Geometry check sheet. Reference: the model listing, model coordinates, mm. A direction names the side the tool comes from. Give positions to 0.01 mm unless a question says otherwise; leave off trailing zeros. Loops run counter-clockwise (first coordinate to the right, second up) from the corner with the lowest first, then second, coordinate; pieces in that order, holes last.
1. Cross-section at C-C, the plane x = 0. Record the cut outline in (y, z).
2. Material ranges on L1, parallel to X at y = 0.9, z = 0; L2, parallel to Z at x = -18.5, y = 0.9; L3, parallel to Y at x = -16, z = -0.5, recorded low to high.
3. Tool access check on faces 1 (the flat face through (-18, 1, 2.5)), 2 (the flat face through (22, 1, 0)), 3 (the flat face through (18, 1, -2.5)). Record the directions out of +Z, -Z, +X, -X, +Y, -Y that give a thin tool (end or side, any length) a straight path to the whole face; none if there is none.
4. Cross-section at A-A, the plane x = -18.5. Record the cut outline in (y, z).
5. Cross-section at D-D, the plane y = 8. Record the cut outline in (x, z).
6. Cross-section at B-B, the plane z = 0. Record the cut outline in (x, y), plus the area to 3 significant figures.
7. Go/stop test with flat-tipped pins: pin 1 Ø3.5 at (x, z) = (-2, -2.5) entering from +Y; pin 2 Ø2 at (x, y) = (-18, 0.5) entering from -Z; pin 3 Ø2 at (x, y) = (17.5, 0.5) entering from +Z. Record where each tip stops, or that it passes through.
8. Release check for a two-part mould opening along Y. For faces 4 (the cylindrical face through (-17.524, 0.986, 0.217)), 5 (the flat face through (0, 19, 0)) record: +Y half, -Y half, draft (parallel to the pull), parting line (faces both ways), or undercut.
from build123d import *

# Parameters (mm, degrees)
SKETCH1_W           = 30
SKETCH1_H           = 30
BOSS_EXTRUDE1_DEPTH = 6
FILLET1_R           = 10
SKETCH3_W           = 7
SKETCH3_H           = 5
SKETCH3_R           = 1
BOSS_EXTRUDE2_DEPTH = 2
FILLET3_R           = 1
SKETCH4_W           = 30
SKETCH4_H           = 30
BOSS_EXTRUDE3_DEPTH = 15
FILLET4_R           = 10
SKETCH5_R           = 5.5
CUT_EXTRUDE2_DEPTH  = 2


with BuildPart() as part:
    # Sketch1 → Boss-Extrude1 (new body)
    with BuildSketch(Plane(origin=(0, 0, 0), x_dir=(1, 0, 0), z_dir=(0, 1, 0))):
        Rectangle(SKETCH1_W, SKETCH1_H)
    extrude(amount=BOSS_EXTRUDE1_DEPTH)

    # Fillet1
    fillet1_edges = [part.edges().sort_by_distance(p)[0] for p in [
        (-15, 3, -15),
        (15, 3, -15),
        (15, 3, 15),
        (-15, 3, 15),
    ]]
    fillet(fillet1_edges, radius=FILLET1_R)

    # Sketch3 → Boss-Extrude2 (add)
    with BuildSketch(Plane.XZ):
        with Locations((18.5, 0)):
            Rectangle(SKETCH3_W, SKETCH3_H)
        with Locations(Location((18.5, 0, 0), (0, 0, 270))):
            Circle(SKETCH3_R, mode=Mode.SUBTRACT)
    boss_extrude2 = extrude(amount=-BOSS_EXTRUDE2_DEPTH)

    # Mirror1: Boss-Extrude2 across plane
    add(boss_extrude2.mirror(Plane(origin=(0, 0, 0), x_dir=(0, 0, 1), z_dir=(1, 0, 0))))

    # Fillet3
    fillet3_edges = [part.edges().sort_by_distance(p)[0] for p in [
        (15, 1, -2.5),
        (15, 1, 2.5),
        (22, 1, 2.5),
        (22, 1, -2.5),
        (-15, 1, 2.5),
        (-15, 1, -2.5),
        (-22, 1, -2.5),
        (-22, 1, 2.5),
    ]]
    fillet(fillet3_edges, radius=FILLET3_R)

    # Sketch4 → Boss-Extrude3 (add)
    with BuildSketch(Plane(origin=(0, 6, 0), x_dir=(1, 0, 0), z_dir=(0, 1, 0))):
        Rectangle(SKETCH4_W, SKETCH4_H)
    extrude(amount=BOSS_EXTRUDE3_DEPTH)

    # Fillet4
    fillet4_edges = [part.edges().sort_by_distance(p)[0] for p in [
        (15, 13.5, 15),
        (15, 13.5, -15),
        (-15, 13.5, -15),
        (-15, 13.5, 15),
    ]]
    fillet(fillet4_edges, radius=FILLET4_R)

    # Sketch5 → Cut-Extrude2 (cut)
    with BuildSketch(Plane(origin=(0, 21, 0), x_dir=(1, 0, 0), z_dir=(0, 1, 0))):
        with Locations(Location((0, 0, 0), (0, 0, 270))):
            Circle(SKETCH5_R)
    extrude(amount=-CUT_EXTRUDE2_DEPTH, mode=Mode.SUBTRACT)


solid = part.part
Result:
1. outline: (0, -15) - (21, -15) - (21, -5.5) - (19, -5.5) - (19, 5.5) - (21, 5.5) - (21, 15) - (0, 15) - close
2. L1: x = -22 to -19.5, -17.5 to 17.5, 19.5 to 22
2. L2: z = -2.5 to -1, 1 to 2.5
2. L3: y = 0 to 2
3. face 1: +Z, -X, +Y, -Y
3. face 2: +Z, -Z, +X, +Y, -Y
3. face 3: -Z, +X, +Y, -Y
4. outline: (0, -2.5) - (2, -2.5) - (2, -1) - (0, -1) - close; (0, 1) - (2, 1) - (2, 2.5) - (0, 2.5) - close
5. outline: (-15, -5) arc R10 ccw to (-5, -15) - (5, -15) arc R10 ccw to (15, -5) - (15, 5) arc R10 ccw to (5, 15) - (-5, 15) arc R10 ccw to (-15, 5) - close
6. outline: (-22, 0) - (-19.5, 0) - (-19.5, 2) - (-22, 2) - close; (-17.5, 0) - (17.5, 0) - (17.5, 2) - (15, 2) - (15, 21) - (5.5, 21) - (5.5, 19) - (-5.5, 19) - (-5.5, 21) - (-15, 21) - (-15, 2) - (-17.5, 2) - close; (19.5, 0) - (22, 0) - (22, 2) - (19.5, 2) - close
6. area: 628 mm2
7. pin 1: stops at y = 19
7. pin 2: stops at z = -2.5
7. pin 3: stops at z = 2.5
8. face 4: draft
8. face 5: +Y half
